from build123d import *

# Parameters (mm, degrees)
F0_W     = 120
F0_H     = 10
F1_DEPTH = 100
F3_DEPTH = 100.001
F4_W     = 10
F4_H     = 10
F5_DEPTH = 70.001


with BuildPart() as f1:
    # F0 (on Front) → F1 (new body)
    with BuildSketch(Plane.XZ):
        with BuildLine():
            Line((-60, 0), (60, 0))
            ThreePointArc((60, 0), (0, 60), (-60, 0))
        make_face()
        with Locations((0, -5)):
            Rectangle(F0_W, F0_H)
    extrude(amount=F1_DEPTH)

    # F2 (on face) → F3 (cut, through all)
    with BuildSketch(Plane.XZ.offset(100)):
        with BuildLine():
            ThreePointArc((35, 0), (43.6443449343, -3.4232659844), (39.6875, 4.9902248196))
            ThreePointArc((39.6875, 4.9902248196), (0, 40), (-39.6875, 4.9902248196))
            ThreePointArc((-39.6875, 4.9902248196), (-43.6443449343, -3.4232659844), (-35, 0))
            Line((-35, 0), (-5, 0))
            ThreePointArc((-5, 0), (0, 5), (5, 0))
            Line((5, 0), (35, 0))
        make_face()
        with BuildLine():
            ThreePointArc((-5, 0), (0, -5), (5, 0))
            Line((5, 0), (-5, 0))
        make_face()
        with BuildLine():
            Line((-5, 0), (5, 0))
            ThreePointArc((5, 0), (0, 5), (-5, 0))
        make_face()
    extrude(amount=-F3_DEPTH, mode=Mode.SUBTRACT)

    # F4 (on face) → F5 (cut, through all)
    with BuildSketch(Plane(origin=(0, 0, -10), x_dir=(1, 0, 0), z_dir=(0, 0, -1))):
        with Locations((-45, 50)):
            Rectangle(F4_W, F4_H)
        with Locations((0, 50)):
            Rectangle(F4_W, F4_H)
        with Locations((45, 50)):
            Rectangle(F4_W, F4_H)
    extrude(amount=-F5_DEPTH, mode=Mode.SUBTRACT)


solid = f1.part
Check sheet for the modelled part. Datum: model origin and axes. Units: mm. A direction names the side the tool comes from. Round coordinates to 2 decimals unless told otherwise and drop trailing zeros. Loops run counter-clockwise (first coordinate to the right, second up) from the corner with the lowest first, then second, coordinate; pieces in that order, holes last. Notation, with made-up numbers: (-36, -2) -> (-15, -2) arc R22 ccw to (-15, 32) -> close; hole circle Ø7 at (66.5, 44). An arc over 180 degrees is marked (long way). Put each result on its own line as item: value. Start each with the question number.
1. Section check B-B (y = -69). Enter the section's corners in (x, z), plus the area to 3 significant figures.
2. Draft check along Y on faces 4 (the face through (-40, -50, 25)), 5 (the face through (-60, -49, -5)), 6 (the face through (-1, 0, 41)), 7 (the face through (0, -55, -7)). Enter one of: +Y half, -Y half, draft (parallel to the pull), parting line (faces both ways), or undercut.
3. Section check A-A (z = 22). Enter the section's corners in (x, y).
4. Section check D-D (z = 29.5). Enter the section's corners in (x, y), plus the area to 3 significant figures.
5. Scan lines: probe 1 along Z at (x, y) = (40, -60); probe 2 along Y at (x, z) = (43, 39); probe 3 along X at (y, z) = (-51, 17). Record each from-to range of solid material in increasing order.
6. Section check C-C (x = -29). Enter the section's corners in (y, z).
7. Gauge pin test, flat ends, axial feed: pin 1 (1 mm diameter, centred on y = -57.5, z = 24, fed in from +X); pin 2 (1.5 mm diameter, centred on x = 22, y = -82.5, fed in from +Z); pin 3 (1.5 mm diameter, centred on x = 29, y = -25.5, fed in from +Z); pin 4 (6 mm diameter, centred on x = 12, z = 34, fed in from +Y). Record the tip position at first contact, or that the pin passes through.
8. Access from +Z, -Z, +X, -X, +Y, -Y to the whole of each face (thin tool, end or side, straight path). Record for faces 1 (the face through (-1, -38, -10)), 2 (the face through (45, -55, 17)), 3 (the face through (0, -23, -5)).
Findings:
1. outline: (-60, -10) -> (60, -10) -> (60, 0) arc R60 ccw to (-60, 0) -> close; hole (-39.69, 4.99) arc R5 ccw (long way) to (-35, 0) -> (-5, 0) arc R5 ccw to (5, 0) -> (35, 0) arc R5 ccw (long way) to (39.69, 4.99) arc R40 ccw to start
1. area: 4,180 mm^2
2. face 4: undercut
2. face 5: draft
2. face 6: +Y half
2. face 7: undercut
3. outline: (-55.82, -100) -> (-33.41, -100) -> (-33.41, 0) -> (-55.82, 0) -> close; (33.41, -100) -> (55.82, -100) -> (55.82, 0) -> (33.41, 0) -> close; hole (-50, -55) -> (-40, -55) -> (-40, -45) -> (-50, -45) -> close; hole (40, -55) -> (50, -55) -> (50, -45) -> (40, -45) -> close
4. outline: (-52.25, -100) -> (-27.01, -100) -> (-27.01, 0) -> (-52.25, 0) -> close; (27.01, -100) -> (52.25, -100) -> (52.25, 0) -> (27.01, 0) -> close; hole (-50, -55) -> (-40, -55) -> (-40, -45) -> (-50, -45) -> close; hole (40, -55) -> (50, -55) -> (50, -45) -> (40, -45) -> close
4. area: 4,850 mm^2
5. probe 1: z = -10 to -5, 5 to 44.72
5. probe 2: y = -100 to -55, -45 to 0
5. probe 3: x = -57.54 to -50, -40 to -36.21, 36.21 to 40, 50 to 57.54
6. outline: (-100, -10) -> (0, -10) -> (0, 0) -> (-100, 0) -> close; (-100, 27.55) -> (0, 27.55) -> (0, 52.53) -> (-100, 52.53) -> close
7. pin 1: stops at x = 55.21
7. pin 2: stops at z = 56.11
7. pin 3: stops at z = 52.93
7. pin 4: passes through
8. face 1: -Z, +X, -X, +Y, -Y
8. face 2: +Z, -Z
8. face 3: +Y, -Y
